```python
from build123d import *
from build123d.topology import SkipClean

# Parameters (mm, degrees)
SKETCH1_R                           = 36.195
SKETCH1_R_2                         = 6.985
BOSS_EXTRUDE1_DEPTH                 = 7.112
BOSS_EXTRUDE2_DEPTH                 = 71.12
CUT_EXTRUDE1_DEPTH                  = 8.128
F_9_64_0_14063_DIAMETER_HOLE2_D     = 3.572002
F_9_64_0_14063_DIAMETER_HOLE2_DEPTH = 5.588
F_9_64_0_14063_DIAMETER_HOLE2_TIP   = 1.073137666


with BuildPart() as part:
    # Sketch1 → Boss-Extrude1 (new body)
    with BuildSketch(Plane(origin=(0, 0, 0), x_dir=(1, 0, 0), z_dir=(0, 1, 0))):
        with Locations(Location((0, 0, 0), (0, 0, 270))):
            Circle(SKETCH1_R)
        with Locations(Location((0, 0, 0), (0, 0, 270))):
            Circle(SKETCH1_R_2, mode=Mode.SUBTRACT)
    extrude(amount=BOSS_EXTRUDE1_DEPTH)

    # Sketch7 → Boss-Extrude2 (add)
    with BuildSketch(Plane(origin=(0, 7.112, 0), x_dir=(1, 0, 0), z_dir=(0, 1, 0))):
        with BuildLine():
            ThreePointArc((5.08, -4.794144866), (0, -6.985), (-5.08, -4.794144866))
            Line((-5.08, -4.794144866), (-5.08, -35.836735691))
            ThreePointArc((-5.08, -35.836735691), (0, -36.195), (5.08, -35.836735691))
            Line((5.08, -35.836735691), (5.08, -4.794144866))
        make_face()
        with BuildLine():
            Line((-5.08, 35.836735691), (-5.08, 4.794144866))
            ThreePointArc((-5.08, 4.794144866), (0, 6.985), (5.08, 4.794144866))
            Line((5.08, 4.794144866), (5.08, 35.836735691))
            ThreePointArc((5.08, 35.836735691), (0, 36.195), (-5.08, 35.836735691))
        make_face()
        with BuildLine():
            Line((-5.08, 4.794144866), (-5.08, 0))
            Line((-5.08, 0), (5.08, 0))
            Line((5.08, 0), (5.08, 4.794144866))
            ThreePointArc((5.08, 4.794144866), (0, 6.985), (-5.08, 4.794144866))
        make_face()
        with BuildLine():
            Line((5.08, 0), (-5.08, 0))
            Line((-5.08, 0), (-5.08, -4.794144866))
            ThreePointArc((-5.08, -4.794144866), (0, -6.985), (5.08, -4.794144866))
            Line((5.08, -4.794144866), (5.08, 0))
        make_face()
    extrude(amount=BOSS_EXTRUDE2_DEPTH)

    # Sketch11 → Cut-Extrude1 (cut)
    with SkipClean():  # the faces are left unmerged after this step: merging them gives an invalid solid
        with BuildSketch(Plane.XZ.offset(-7.112)):
            with BuildLine():
                Line((-5.08, 4.794144866), (-5.08, -4.794144866))
                ThreePointArc((-5.08, -4.794144866), (0, -6.985), (5.08, -4.794144866))
                Line((5.08, -4.794144866), (5.08, 4.794144866))
                ThreePointArc((5.08, 4.794144866), (0, 6.985), (-5.08, 4.794144866))
            make_face()
        extrude(amount=-CUT_EXTRUDE1_DEPTH, mode=Mode.SUBTRACT)

    # 9/64 (0.14063) Diameter Hole2
    with Locations(Plane(origin=(0, 0, 0), x_dir=(-1, 0, 0), z_dir=(0, -1, 0))):
        with Locations((-19.05, 0), (19.05, 0)):
            Hole(F_9_64_0_14063_DIAMETER_HOLE2_D / 2, depth=F_9_64_0_14063_DIAMETER_HOLE2_DEPTH)
            with Locations((0, 0, -(F_9_64_0_14063_DIAMETER_HOLE2_DEPTH + F_9_64_0_14063_DIAMETER_HOLE2_TIP / 2))):  # 118° drill point
                Cone(0, F_9_64_0_14063_DIAMETER_HOLE2_D / 2, F_9_64_0_14063_DIAMETER_HOLE2_TIP, mode=Mode.SUBTRACT)


solid = part.part
```
CAD build for the part. Positions are in the model's coordinates, mm. A direction names the side the tool comes from. Coordinates: 2 decimals unless noted, no trailing zeros. Order: outer loops, then holes, each group sorted by start corner. A loop starts at its lowest first (then second) coordinate and runs counter-clockwise, first axis right, second up. Notation, with made-up numbers: (29, 44.5) - (37, 44.5) arc R16 ccw to (37, 72.5) - close; hole circle Ø6 at (25, -27.75). An arc over 180 degrees is marked (long way). Answer in a Markdown table with one row per item.
1. Slice it at C-C, the plane y = 39.5. List the corners of the cut face in (x, z) (3 decimals), then the cut area to 3 significant figures.
Answer:
| item | result |
|---|---|
| outline | (-5.08, -35.837) arc R36.195 ccw to (5.08, -35.837) - (5.08, 35.837) arc R36.195 ccw to (-5.08, 35.837) - close |
| area | 733 mm² |
2. Slice it at B-B, the plane z = 19. List the corners of the cut face in (x, y), then the cut area to 3 significant figures.
Answer:
| item | result |
|---|---|
| outline | (-30.81, 0) - (30.81, 0) - (30.81, 7.11) - (5.08, 7.11) - (5.08, 78.23) - (-5.08, 78.23) - (-5.08, 7.11) - (-30.81, 7.11) - close |
| area | 1,160 mm² |
3. 3-axis set-ups, long thin cutter, end or side, ignore diameter. For faces 1 (the face through (17, 7.112, -1)), 2 (the face through (-17, 7.112, -1)), 3 (the face through (-8, 0, -1)), 4 (the face through (-1.33, 24.45, 36.17)), 5 (the face through (-20.834, 2.833, -0.079)): which of +Z, -Z, +X, -X, +Y, -Y reach the whole face in a straight line?
Answer:
| item | result |
|---|---|
| face 1 | +Z, -Z, +X, +Y |
| face 2 | +Z, -Z, -X, +Y |
| face 3 | +Z, -Z, +X, -X, -Y |
| face 4 | +Y, -Y |
| face 5 | -Y |
4. Slice it at D-D, the plane x = 12.5. List the corners of the cut face in (y, z).
Answer:
| item | result |
|---|---|
| outline | (0, -33.97) - (7.11, -33.97) - (7.11, 33.97) - (0, 33.97) - close |
5. Slice it at A-A, the plane x = 0. List the corners of the cut face in (y, z) (3 decimals), then the cut area to 3 significant figures.
Answer:
| item | result |
|---|---|
| outline | (0, -36.195) - (78.232, -36.195) - (78.232, 36.195) - (0, 36.195) - (0, 6.985) - (15.24, 6.985) - (15.24, -6.985) - (0, -6.985) - close |
| area | 5,450 mm² |
6. Pull direction X, two halves, no side cores. Call faces 6 (the face through (0, 78.232, -1)), 7 (the face through (18.8, 6.5, -0.1)), 8 (the face through (5.08, 42, 1)): +X half, -X half, draft (parallel to the pull), parting line (faces both ways), or undercut.
Answer:
| item | result |
|---|---|
| face 6 | draft |
| face 7 | undercut |
| face 8 | +X half |
7. Flat gauge pins, fed straight in: P1, Ø5, axis at x = -0.5, z = -3, coming from the -Y side; P2, Ø1.5, axis at x = -7.5, y = 47, coming from the -Z side; P3, Ø9.5, axis at x = 20, z = 2.5, coming from the +Y side; P4, Ø4, axis at y = 11.5, z = -4.5, coming from the -X side. Where does each tip first touch, or does it go through?
Answer:
| item | result |
|---|---|
| P1 | y = 15.24 |
| P2 | through |
| P3 | y = 7.11 |
| P4 | x = -5.08 |
8. Drill centre lines: L1, parallel to X at y = 15.5, z = -4.5; L2, parallel to Y at x = -5.5, z = 16; L3, parallel to Z at x = 0, y = 4.25 (3 decimals). Where is each one in solid material? Low to high. Write a range as from..to.
Answer:
| item | result |
|---|---|
| L1 | -5.08..5.08 |
| L2 | 0..7.11 |
| L3 | -36.195..-6.985, 6.985..36.195 |
